from build123d import *

# Parameters (mm, degrees)
BOSS_EXTRUDE1_DEPTH = 20
SKETCH2_R           = 1.5
BOSS_EXTRUDE2_DEPTH = 5
CUT_EXTRUDE1_START  = -20
SKETCH2_2_R         = 1.5
CUT_EXTRUDE1_DEPTH  = 5


with BuildPart() as part:
    # Sketch1 → Boss-Extrude1 (new body)
    with BuildSketch(Plane(origin=(0, 0, 0), x_dir=(1, 0, 0), z_dir=(0, 1, 0))):
        Polygon((2.598076211, 0), (1.299038106, 2.25), (-1.299038106, 2.25), (-2.598076211, 0), (-1.299038106, -2.25), (1.299038106, -2.25), align=None)
    extrude(amount=BOSS_EXTRUDE1_DEPTH)

    # Sketch2 → Boss-Extrude2 (add)
    with BuildSketch(Plane.XZ):
        Circle(SKETCH2_R)
    extrude(amount=BOSS_EXTRUDE2_DEPTH)

    # Sketch2<2> → Cut-Extrude1 (cut)
    with BuildSketch(Plane.XZ.offset(CUT_EXTRUDE1_START)):
        Circle(SKETCH2_2_R)
    extrude(amount=CUT_EXTRUDE1_DEPTH, mode=Mode.SUBTRACT)


solid = part.part
Input: part model. Units: mm. Frame: model coordinates. A direction names the side the tool comes from. Give positions to 0.01 mm unless a question says otherwise; leave off trailing zeros. Order: outer loops, then holes, each group sorted by start corner. A loop starts at its lowest first (then second) coordinate and runs counter-clockwise, first axis right, second up. Notation, with made-up numbers: (-34, 70) -> (25, 70) arc R23 ccw to (25, 83) -> close; hole circle Ø6 at (-27.75, -0.5). An arc over 180 degrees is marked (long way). Use one line per item in the form item = value.
1) Section A-A, the plane x = 0. Return loops of the section in (y, z).
Response values:
outline = (-5, -1.5) -> (0, -1.5) -> (0, -2.25) -> (20, -2.25) -> (20, -1.5) -> (15, -1.5) -> (15, 1.5) -> (20, 1.5) -> (20, 2.25) -> (0, 2.25) -> (0, 1.5) -> (-5, 1.5) -> close
2) Section B-B, the plane y = 17. Return loops of the section in (x, z), and give its area (3 significant figures).
Response values:
outline = (-2.6, 0) -> (-1.3, -2.25) -> (1.3, -2.25) -> (2.6, 0) -> (1.3, 2.25) -> (-1.3, 2.25) -> close; hole circle Ø3 at (0, 0)
area = 10.5 mm^2
3) Section C-C, the plane z = -0.35. Return loops of the section in (x, y), and give its area (3 significant figures).
Response values:
outline = (-2.4, 0) -> (-1.46, 0) -> (-1.46, -5) -> (1.46, -5) -> (1.46, 0) -> (2.4, 0) -> (2.4, 20) -> (1.46, 20) -> (1.46, 15) -> (-1.46, 15) -> (-1.46, 20) -> (-2.4, 20) -> close
area = 95.8 mm^2
4) Section D-D, the plane y = -2.75. Return loops of the section in (x, z), and give its area (3 significant figures).
Response values:
outline = circle Ø3 at (0, 0)
area = 7.07 mm^2
5) Mould query, pull axis X, two halves, no side actions, for faces 1 (the flat face through (1.958, 9.86, -1.109)), 2 (the flat face through (0, 0, -2)), 3 (the cylindrical face through (-1.5, 17.54, 0.07)). Classes: pulls with the +X half, pulls with the -X half, needs draft (parallel to the pull), parting line crosses it, or undercut.
Response values:
face_1 = pulls with the +X half
face_2 = needs draft
face_3 = undercut
6) First-contact query: pin 1 Ø0.9 at (x, z) = (-0.5, 0) entering from +Y. Flat tip, straight axial feed; report the tip coordinate or a pass-through.
Response values:
pin_1 = 15
7) Reachability of faces 4 (the cylindrical face through (-1.5, -2.46, 0.07)), 5 (the flat face through (0, 10, 2.25)), 6 (the flat face through (0, 15, 0)) from +Z, -Z, +X, -X, +Y, -Y: full face, straight path, thin tool, end or side. Return the list, or none.
Response values:
face_4 = -Y
face_5 = +Z, +X, -X, +Y, -Y
face_6 = +Y
8) Line query: probe 1 along Z at (x, y) = (0, 16.3); probe 2 along Y at (x, z) = (-1.3, 1.1); probe 3 along Y at (x, z) = (0.1, 0.1). Output: solid intervals per line, ascending.
Response values:
probe_1 = -2.25 to -1.5, 1.5 to 2.25
probe_2 = 0 to 20
probe_3 = -5 to 15
